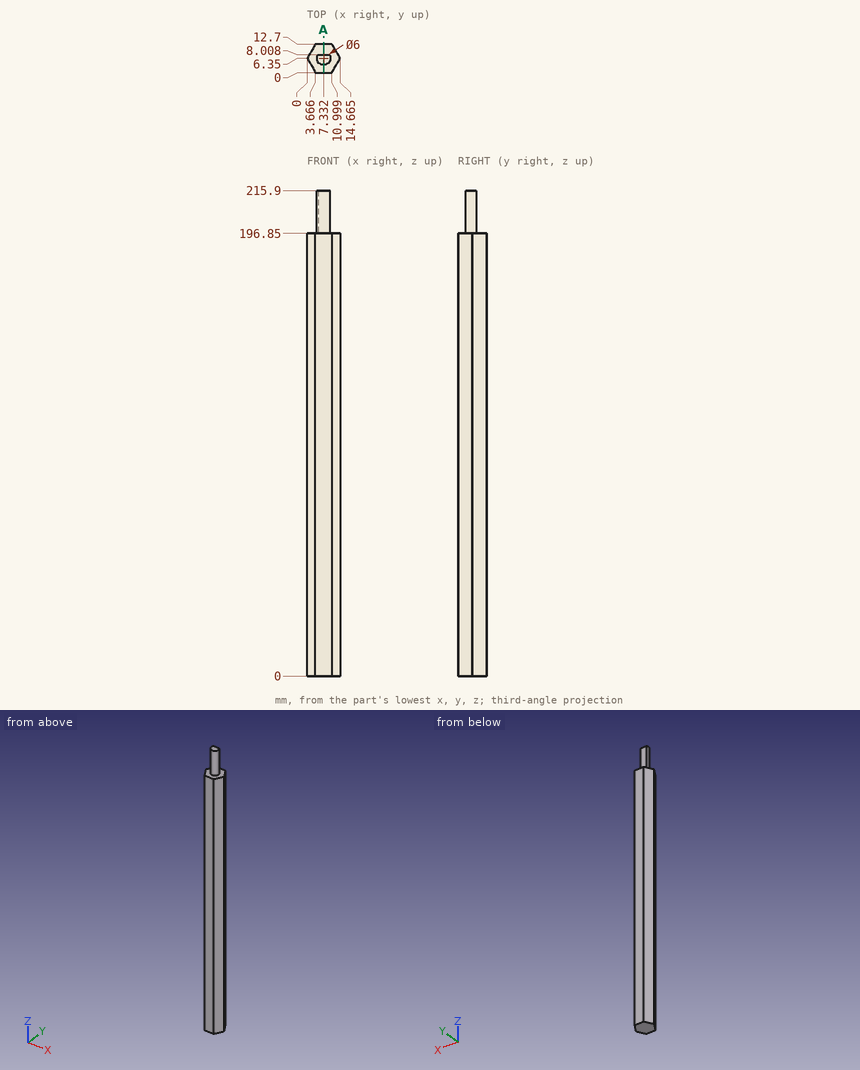
Check sheet for the drawn part. Datum: minimum x, y, z corner. Units: mm. Round coordinates to 2 decimals unless told otherwise and drop trailing zeros. Order: outer loops, then holes, each group sorted by start corner. A loop starts at its lowest first (then second) coordinate and runs counter-clockwise, first axis right, second up. Notation, with made-up numbers: (22.25, 73) -> (54.25, 73) arc R10 ccw to (54.25, 87) -> close; hole circle Ø10 at (63.5, -29.5). An arc over 180 degrees is marked (long way). Put each result on its own line as item: value.
1) Material ranges on line 1 (Z direction, x = 10.5, y = 6.25); line 2 (X direction, y = 6, z = 205); line 3 (X direction, y = 4.75, z = 27) (1 decimal), recorded low to high.
Final values:
line 1: z = 0 to 196.85
line 2: x = 4.35 to 10.31
line 3: x = 0.9 to 13.7
2) Section check A-A (x = 7.25). Record the cut outline in (y, z).
Final values:
outline: (0, 0) -> (12.7, 0) -> (12.7, 196.85) -> (8.01, 196.85) -> (8.01, 215.9) -> (3.35, 215.9) -> (3.35, 196.85) -> (0, 196.85) -> close
3) Depth check by flat-ended pin: pin 1 (4 mm diameter, centred on y = 3, z = 23, fed in from +X) (1 decimal); pin 2 (1.5 mm diameter, centred on x = 7.5, z = 206, fed in from +Y); pin 3 (5 mm diameter, centred on y = 11.5, z = 179, fed in from +X) (1 decimal). Enter the tip coordinate at first touch or a pass-through.
Final values:
pin 1: stops at x = 13.9
pin 2: stops at y = 8.01
pin 3: stops at x = 13.1
